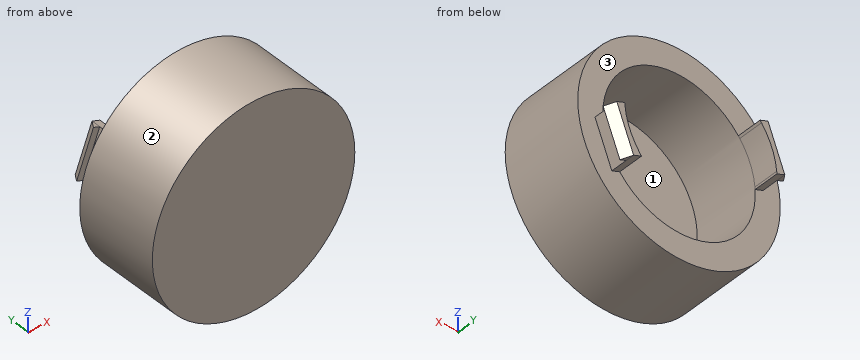
```python
from build123d import *

# Parameters (mm, degrees)
SKETCH1_R            = 15.24
BOSS_EXTRUDE1_DEPTH  = 12.7
BOSS_EXTRUDE10_DEPTH = 3.81
BOSS_EXTRUDE11_DEPTH = 6.989290822
BOSS_EXTRUDE12_DEPTH = 6.985
SKETCH9_R            = 11.477020293
CUT_EXTRUDE3_DEPTH   = 10.16


with BuildPart() as part:
    # Sketch1 → Boss-Extrude1 (new body)
    with BuildSketch(Plane(origin=(0, 0, 0), x_dir=(1, 0, 0), z_dir=(0, 1, 0))):
        Circle(SKETCH1_R)
    extrude(amount=BOSS_EXTRUDE1_DEPTH)

    # Sketch3 → Boss-Extrude10 (add)
    with BuildSketch(Plane(origin=(0, 12.7, 0), x_dir=(1, 0, 0), z_dir=(0, 1, 0))):
        with BuildLine():
            Line((11.427775698, 1.062043977), (12.64550795, 1.175214312))
            Line((12.64550795, 1.175214312), (10.116961472, 7.677049601))
            Line((10.116961472, 7.677049601), (9.142722214, 6.937768036))
            ThreePointArc((9.142722214, 6.937768036), (10.696605975, 4.159881659), (11.427775698, 1.062043977))
        make_face()
        with BuildLine():
            Line((9.142722214, 6.937768036), (10.116961472, 7.677049601))
            Line((10.116961472, 7.677049601), (8.93331892, 7.216734155))
            Line((8.93331892, 7.216734155), (8.94183947, 7.194824647))
            ThreePointArc((8.94183947, 7.194824647), (9.043194256, 7.06701015), (9.142722214, 6.937768036))
        make_face()
        with BuildLine():
            Line((11.461865398, 0.714898867), (12.64550795, 1.175214312))
            Line((12.64550795, 1.175214312), (11.427775698, 1.062043977))
            ThreePointArc((11.427775698, 1.062043977), (11.441715952, 0.899517032), (11.453344849, 0.736808375))
            Line((11.453344849, 0.736808375), (11.461865398, 0.714898867))
        make_face()
        with BuildLine():
            Line((-9.142722214, -6.937768036), (-10.116961472, -7.677049601))
            Line((-10.116961472, -7.677049601), (-8.926355488, -7.214026095))
            ThreePointArc((-8.926355488, -7.214026095), (-9.035594717, -7.076724025), (-9.142722214, -6.937768036))
        make_face()
        with BuildLine():
            Line((-11.427775698, -1.062043977), (-12.64550795, -1.175214312))
            Line((-12.64550795, -1.175214312), (-10.116961472, -7.677049601))
            Line((-10.116961472, -7.677049601), (-9.142722214, -6.937768036))
            ThreePointArc((-9.142722214, -6.937768036), (-10.696605975, -4.159881659), (-11.427775698, -1.062043977))
        make_face()
        with BuildLine():
            Line((-11.454901967, -0.712190807), (-12.64550795, -1.175214312))
            Line((-12.64550795, -1.175214312), (-11.427775698, -1.062043977))
            ThreePointArc((-11.427775698, -1.062043977), (-11.44267598, -0.887221069), (-11.454901967, -0.712190807))
        make_face()
    extrude(amount=BOSS_EXTRUDE10_DEPTH)

    # Sketch6 → Boss-Extrude11 (add)
    with BuildSketch(Plane(origin=(-1.264273239, 0, -3.250917644), x_dir=(-0.932002009, 0, 0.362453107), z_dir=(-0.362453107, 0, -0.932002009))):
        Polygon((12.211598898, 16.51), (12.211598898, 15.157865498), (13.227598898, 15.157865498), align=None)
    extrude(amount=-BOSS_EXTRUDE11_DEPTH)

    # Sketch7 → Boss-Extrude12 (add)
    with BuildSketch(Plane(origin=(1.264273239, 0, 3.250917644), x_dir=(0.932002009, 0, -0.362453107), z_dir=(0.362453107, 0, 0.932002009))):
        Polygon((12.211598898, 16.51), (12.211598898, 15.207573147), (13.227598898, 15.207573147), align=None)
    extrude(amount=-BOSS_EXTRUDE12_DEPTH)

    # Sketch9 → Cut-Extrude3 (cut)
    with BuildSketch(Plane(origin=(0, 12.7, 0), x_dir=(1, 0, 0), z_dir=(0, 1, 0))):
        Circle(SKETCH9_R)
    extrude(amount=-CUT_EXTRUDE3_DEPTH, mode=Mode.SUBTRACT)


solid = part.part
```
Work out the finished part from the listing and answer in its coordinate system (mm). Face numbers are marked on the shaded views. Round coordinates to 2 decimals unless told otherwise and drop trailing zeros. Loops run counter-clockwise (first coordinate to the right, second up) from the corner with the lowest first, then second, coordinate; pieces in that order, holes last.
(1) Each of these flat-tipped pins is pushed along its axis until it touches: P1, Ø5, axis at x = -10.5, z = -10.5, coming from the -Y side; P2, Ø2, axis at x = 1.5, y = 2, coming from the +Z side; P3, Ø5, axis at x = 2.5, z = 10, coming from the +Y side; P4, Ø3, axis at y = 2.5, z = 2, coming from the -X side. Where does it stop, or does it pass through?
Computed values:
P1: stops at y = 0
P2: stops at z = 15.23
P3: stops at y = 12.7
P4: stops at x = -15.23
(2) Find the intervals of material crossed by L1, parallel to Z at x = 0, y = 10.25; L2, parallel to Y at x = 7.5, z = -7, in increasing order.
Computed values:
L1: z = -15.24 to -11.48, 11.48 to 15.24
L2: y = 0 to 2.54
(3) The part is cut by section C-C, the plane y = 11. Give the vertices of the cut face in (x, z).
Computed values:
outline: circle Ø30.48 at (0, 0); hole circle Ø22.95 at (0, 0)
(4) The mould has two halves that part along Z. Classify the marked faces 1, 2 and 3: pulls with the +Z half, pulls with the -Z half, needs draft (parallel to the pull), parting line crosses it, or undercut.
Computed values:
face 1: undercut
face 2: parting line crosses it
face 3: needs draft
(5) The part is cut by section B-B, the plane z = 0. Give the vertices of the cut face in (x, y).
Computed values:
outline: (-15.24, 0) - (15.24, 0) - (15.24, 12.7) - (11.48, 12.7) - (11.48, 2.54) - (-11.48, 2.54) - (-11.48, 12.7) - (-15.24, 12.7) - close
(6) The part is cut by section D-D, the plane z = -3.5. Give the vertices of the cut face in (x, y), and give its area (3 significant figures).
Computed values:
outline: (-14.83, 0) - (14.83, 0) - (14.83, 12.7) - (11.74, 12.7) - (11.74, 15.21) - (12.83, 15.21) - (11.74, 16.51) - (10.93, 16.51) - (10.93, 2.54) - (-10.93, 2.54) - (-10.93, 12.7) - (-14.83, 12.7) - close
area: 158 mm2
(7) The part is cut by section A-A, the plane x = 0. Give the vertices of the cut face in (y, z), and give its area (3 significant figures).
Computed values:
outline: (0, -15.24) - (12.7, -15.24) - (12.7, -11.48) - (2.54, -11.48) - (2.54, 11.48) - (12.7, 11.48) - (12.7, 15.24) - (0, 15.24) - close
area: 154 mm2
